from build123d import *

# Parameters (mm, degrees)
F1_DEPTH = 25.4


with BuildPart() as f1:
    # F0 (on Front) → F1 (new body)
    with BuildSketch(Plane.XZ):
        Polygon((88.974215, 65.948948), (54.8627, 65.948948), (54.8627, 58.892507), (54.8627, 48.893191), (88.974215, 48.893191), align=None)
        with BuildLine():
            Line((19.848254, 12.507557), (35.532828, 12.507557))
            Line((35.532828, 12.507557), (35.532828, 30.700376))
            ThreePointArc((35.532828, 30.700376), (40.023166, 40.382017), (50.314497, 43.207932))
            Line((50.314497, 43.207932), (86.637879, 43.207932))
            Line((86.637879, 43.207932), (88.974215, 48.893191))
            Line((88.974215, 48.893191), (54.8627, 48.893191))
            Line((54.8627, 48.893191), (54.8627, 58.892507))
            Line((54.8627, 58.892507), (51.360797, 58.892507))
            ThreePointArc((51.360797, 58.892507), (29.301535, 51.841785), (19.848254, 30.700376))
            Line((19.848254, 30.700376), (19.848254, 12.507557))
        make_face()
        with BuildLine():
            add(Edge.make_bspline(
                [(-35.532828, 12.507557), (-19.614134, 45.482036), (19.045593, 66.51748), (54.8627, 65.948948)],
                knots=[0, 0, 0, 0, 105.011113, 105.011113, 105.011113, 105.011113], degree=3))
            Line((-35.532828, 12.507557), (19.848254, 12.507557))
            Line((19.848254, 12.507557), (19.848254, 30.700376))
            ThreePointArc((19.848254, 30.700376), (29.301535, 51.841785), (51.360797, 58.892507))
            Line((51.360797, 58.892507), (54.8627, 58.892507))
            Line((54.8627, 58.892507), (54.8627, 65.948948))
        make_face()
        Polygon((-35.532828, -12.507557), (35.532828, -12.507557), (35.532828, 12.507557), (19.848254, 12.507557), (-35.532828, 12.507557), align=None)
    extrude(amount=F1_DEPTH)


solid = f1.part
Read the model definition and answer for the solid it produces. Units are mm, in the model's axes. A direction names the side the tool comes from. Give positions to 0.01 mm unless a question says otherwise; leave off trailing zeros. Write each loop counter-clockwise with the first axis right and the second up, starting at its lowest first coordinate (ties: lowest second). Pieces come first, ordered by that corner, then holes. Notation, with made-up numbers: (9, 7) - (26, 7) arc R17 ccw to (26, 14) - close; hole circle Ø7 at (-36.75, 1). An arc over 180 degrees is marked (long way). Answer in a Markdown table with one row per item. Add a question column.
Item 1: A tool of negligible diameter and unlimited length cuts with its end or side. For faces 1 (the face through (-35.533, -13, 0)), 2 (the face through (68, -13, 43.208)), from which of +Z, -Z, +X, -X, +Y, -Y can it reach the whole face along a straight path? Write none if from no direction.
Item 2: Find the intervals of material crossed by L1, parallel to Z at x = 66.5, y = -2; L2, parallel to X at y = -18.25, z = 9; L3, parallel to Z at x = 17, y = -11.25, in increasing order.
Item 3: Determine the mould class of faces 3 (the face through (39.906, -12.522, 40.282)), 4 (the face through (87.79, -12.52, 46.01)), 5 (the face through (12, -25.4, 28)) for opening direction X: pulls with the +X half, pulls with the -X half, needs draft (parallel to the pull), parting line crosses it, or undercut.
Item 4: Flat-ended cylindrical pins translate along their axes: P1, Ø1.5, axis at y = -16.5, z = 22, coming from the -X side; P2, Ø1.5, axis at x = 42.5, y = -21.5, coming from the +Z side; P3, Ø1.5, axis at y = -10, z = 42, coming from the -X side. Find the tip coordinate at first contact, or state that the pin passes through.
Item 5: Section A-A, the plane z = 7 is taken. Write down the section's boundary in (x, y), and give its area (3 significant figures).
Recorded:
| question | item | result |
|---|---|---|
| 1 | face 1 | +Z, -Z, -X, +Y, -Y |
| 1 | face 2 | -Z, +X, +Y, -Y |
| 2 | L1 | z = 43.21 to 65.95 |
| 2 | L2 | x = -35.53 to 35.53 |
| 2 | L3 | z = -12.51 to 58.9 |
| 3 | face 3 | undercut |
| 3 | face 4 | pulls with the +X half |
| 3 | face 5 | needs draft |
| 4 | P1 | stops at x = -30.61 |
| 4 | P2 | stops at z = 65.4 |
| 4 | P3 | stops at x = -12.86 |
| 5 | outline | (-35.53, -25.4) - (35.53, -25.4) - (35.53, 0) - (-35.53, 0) - close |
| 5 | area | 1,810 mm2 |
